Check sheet for the modelled part. Datum: model origin and axes. Units: mm. A direction names the side the tool comes from. Give positions to 0.01 mm unless a question says otherwise; leave off trailing zeros. Write each loop counter-clockwise with the first axis right and the second up, starting at its lowest first coordinate (ties: lowest second). Pieces come first, ordered by that corner, then holes. Notation, with made-up numbers: M -31,71.5 L -14,71.5 A17 ccw -14,78.5 Z; hole C 29.5,30.5 d6. An arc over 180 degrees is marked long. Use CSV: the item, a comma, the result in double quotes. Start each with the question number.
1. Scan lines: line 1 (Y direction, x = 6, z = 48); line 2 (X direction, y = 0, z = 40.5). Record each from-to range of solid material in increasing order.
2. Depth check by flat-ended pin: P1, Ø6, axis at x = -1, z = 45, coming from the -Y side; P2, Ø12, axis at y = 1, z = 43, coming from the +X side; P3, Ø2.5, axis at x = -1, z = 30.5, coming from the -Y side; P4, Ø0.5, axis at x = -4, z = 28.5, coming from the -Y side. Enter the tip coordinate at first touch or a pass-through.
3. Cross-section at A-A, the plane x = -6.5. Enter the section's corners in (y, z).
4. Mould release check, pull along Y, two halves, no side actions. Record for faces 5 (the face through (7, 10, 30)), 6 (the face through (9.15, 8, 30)), 7 (the face through (0, -3, 50)): +Y half, -Y half, draft (parallel to the pull), parting line (faces both ways), or undercut.
5. Access from +Z, -Z, +X, -X, +Y, -Y to the whole of each face (thin tool, end or side, straight path). Record for faces 1 (the face through (-3.967, -9.051, 29.72)), 2 (the face through (-9.051, -3.967, 29.72)), 3 (the face through (4.67, 3.82, 29.72)), 4 (the face through (-10, 7, 30)).
6. Cross-section at D-D, the plane z = 14. State how many separate pieces and enclosed holes the cut face has, and give its area (3 significant figures).
7. Cross-section at B-B, the plane y = 0. Enter the section's corners in (x, z).
Autodesk Inventor part; units mm, degrees
ref_plane "Начальная плоскость" through (0, 0, 10) normal (0, 0, 1) x (1, 0, 0)
ref_plane "Конечная плоскость" through (0, 0, 50) normal (0, 0, 1) x (1, 0, 0)
ref_plane "РабПлоскость4" through (-8.5, 255, 50) normal (0, 0, 1) x (1, 0, 0)
ref_plane "Начальная плоскость" through (0, 0, 10) normal (0, 0, 1) x (1, 0, 0)
ref_plane "Конечная плоскость" through (0, 0, 50) normal (0, 0, 1) x (1, 0, 0)
sketch "Эскиз" plane through (0, 0, 0) normal (0, 0, 1) x (1, 0, 0)
  line L0 (-14.4349, 0) -> (14.4349, 0)
  line L1 (0, -14) -> (0, 14)
  line L2 (0, 0) -> (7.5, 7.5) construction
  circle A0 centre (7.5, 7.5) radius 1.65 construction
  line L3 (5.85, 9.15) -> (9.15, 9.15)
  line L4 (9.15, 9.15) -> (9.15, 5.85)
  line L5 (9.15, 5.85) -> (5.85, 5.85)
  line L6 (5.85, 5.85) -> (5.85, 9.15)
  line L7 (3.235, 8.1636) -> (4.72, 9.9636)
  line L8 (4.7971, 10) -> (8.5, 10)
  line L9 (3.3121, 8) -> (4.95, 8)
  line L10 (4.95, 8) -> (4.95, 5.7985)
  line L11 (4.95, 5.7985) -> (2.6515, 3.5)
  line L12 (0, 3.5) -> (2.6515, 3.5)
  circle A1 centre (0, 0) radius 2.5
  line L13 (8.1636, 3.235) -> (9.9636, 4.72)
  line L14 (10, 4.7971) -> (10, 8.5)
  line L15 (8, 3.3121) -> (8, 4.95)
  line L16 (8, 4.95) -> (5.7985, 4.95)
  line L17 (5.7985, 4.95) -> (3.5, 2.6515)
  line L18 (3.5, 0) -> (3.5, 2.6515)
  arc A2 (10, 8.5) -> (8.5, 10) centre (8.5, 8.5) ccw
  line L19 (0, 0) -> (-7.5, 7.5) construction
  circle A3 centre (-7.5, 7.5) radius 1.65 construction
  line L20 (-5.85, 9.15) -> (-9.15, 9.15)
  line L21 (-9.15, 9.15) -> (-9.15, 5.85)
  line L22 (-9.15, 5.85) -> (-5.85, 5.85)
  line L23 (-5.85, 5.85) -> (-5.85, 9.15)
  line L24 (-3.235, 8.1636) -> (-4.72, 9.9636)
  line L25 (-4.7971, 10) -> (-8.5, 10)
  line L26 (-3.3121, 8) -> (-4.95, 8)
  line L27 (-4.95, 8) -> (-4.95, 5.7985)
  line L28 (-4.95, 5.7985) -> (-2.6515, 3.5)
  line L29 (0, 3.5) -> (-2.6515, 3.5)
  line L30 (-3.5, 0) -> (-3.5, 2.6515)
  line L31 (-5.7985, 4.95) -> (-3.5, 2.6515)
  line L32 (-8, 4.95) -> (-5.7985, 4.95)
  line L33 (-8, 3.3121) -> (-8, 4.95)
  line L34 (-8.1636, 3.235) -> (-9.9636, 4.72)
  line L35 (-10, 4.7971) -> (-10, 8.5)
  arc A4 (-8.5, 10) -> (-10, 8.5) centre (-8.5, 8.5) ccw
  line L36 (0, 14) -> (0, -14)
  line L37 (0, 0) -> (7.5, -7.5) construction
  circle A5 centre (7.5, -7.5) radius 1.65 construction
  line L38 (5.85, -9.15) -> (9.15, -9.15)
  line L39 (9.15, -9.15) -> (9.15, -5.85)
  line L40 (9.15, -5.85) -> (5.85, -5.85)
  line L41 (5.85, -5.85) -> (5.85, -9.15)
  line L42 (3.235, -8.1636) -> (4.72, -9.9636)
  line L43 (4.7971, -10) -> (8.5, -10)
  line L44 (3.3121, -8) -> (4.95, -8)
  line L45 (4.95, -8) -> (4.95, -5.7985)
  line L46 (4.95, -5.7985) -> (2.6515, -3.5)
  line L47 (0, -3.5) -> (2.6515, -3.5)
  line L48 (3.5, 0) -> (3.5, -2.6515)
  line L49 (5.7985, -4.95) -> (3.5, -2.6515)
  line L50 (8, -4.95) -> (5.7985, -4.95)
  line L51 (8, -3.3121) -> (8, -4.95)
  line L52 (8.1636, -3.235) -> (9.9636, -4.72)
  line L53 (10, -4.7971) -> (10, -8.5)
  arc A6 (8.5, -10) -> (10, -8.5) centre (8.5, -8.5) ccw
  line L54 (0, 0) -> (-7.5, -7.5) construction
  line L55 (-4.95, -8) -> (-4.95, -5.7985)
  line L56 (-3.3121, -8) -> (-4.95, -8)
  line L57 (-5.7985, -4.95) -> (-3.5, -2.6515)
  line L58 (-4.95, -5.7985) -> (-2.6515, -3.5)
  line L59 (-3.5, 0) -> (-3.5, -2.6515)
  line L60 (0, -3.5) -> (-2.6515, -3.5)
  circle A7 centre (-7.5, -7.5) radius 1.65 construction
  line L61 (-5.85, -5.85) -> (-5.85, -9.15)
  line L62 (-5.85, -9.15) -> (-9.15, -9.15)
  line L63 (-9.15, -9.15) -> (-9.15, -5.85)
  line L64 (-9.15, -5.85) -> (-5.85, -5.85)
  line L65 (-3.235, -8.1636) -> (-4.72, -9.9636)
  line L66 (-8, -4.95) -> (-5.7985, -4.95)
  line L67 (-8, -3.3121) -> (-8, -4.95)
  line L68 (-8.1636, -3.235) -> (-9.9636, -4.72)
  line L69 (-4.7971, -10) -> (-8.5, -10)
  line L70 (-10, -4.7971) -> (-10, -8.5)
  arc A8 (-10, -8.5) -> (-8.5, -10) centre (-8.5, -8.5) ccw
  arc A9 (3.235, 8.1636) -> (3.3121, 8) centre (3.3121, 8.1) ccw
  arc A10 (4.7971, 10) -> (4.72, 9.9636) centre (4.7971, 9.9) ccw
  arc A11 (8, 3.3121) -> (8.1636, 3.235) centre (8.1, 3.3121) ccw
  arc A12 (9.9636, 4.72) -> (10, 4.7971) centre (9.9, 4.7971) ccw
  arc A13 (-3.3121, 8) -> (-3.235, 8.1636) centre (-3.3121, 8.1) ccw
  arc A14 (-4.72, 9.9636) -> (-4.7971, 10) centre (-4.7971, 9.9) ccw
  arc A15 (-8.1636, 3.235) -> (-8, 3.3121) centre (-8.1, 3.3121) ccw
  arc A16 (-10, 4.7971) -> (-9.9636, 4.72) centre (-9.9, 4.7971) ccw
  arc A17 (-8, -3.3121) -> (-8.1636, -3.235) centre (-8.1, -3.3121) ccw
  arc A18 (-9.9636, -4.72) -> (-10, -4.7971) centre (-9.9, -4.7971) ccw
  arc A19 (-3.235, -8.1636) -> (-3.3121, -8) centre (-3.3121, -8.1) ccw
  arc A20 (-4.7971, -10) -> (-4.72, -9.9636) centre (-4.7971, -9.9) ccw
  arc A21 (4.72, -9.9636) -> (4.7971, -10) centre (4.7971, -9.9) ccw
  arc A22 (3.3121, -8) -> (3.235, -8.1636) centre (3.3121, -8.1) ccw
  arc A23 (8.1636, -3.235) -> (8, -3.3121) centre (8.1, -3.3121) ccw
  arc A24 (10, -4.7971) -> (9.9636, -4.72) centre (9.9, -4.7971) ccw
  point P0 (3.1, 8)
  point P1 (4.75, 10)
  point P2 (7.5, 9.15)
  point P3 (8, 3.1)
  point P4 (10, 4.75)
  point P5 (7.5, 5.85)
  point P6 (9.15, 7.5)
  point P7 (-3.1, 8)
  point P8 (-4.75, 10)
  point P9 (-7.5, 9.15)
  point P10 (-8, 3.1)
  point P11 (-10, 4.75)
  point P12 (-7.5, 5.85)
  point P13 (-9.15, 7.5)
  point P14 (3.1, -8)
  point P15 (4.75, -10)
  point P16 (7.5, -9.15)
  point P17 (8, -3.1)
  point P18 (10, -4.75)
  point P19 (7.5, -5.85)
  point P20 (9.15, -7.5)
  point P21 (-3.1, -8)
  point P22 (-7.5, -5.85)
  point P23 (-7.5, -9.15)
  point P24 (-9.15, -7.5)
  point P25 (-4.75, -10)
  point P26 (-8, -3.1)
  point P27 (-10, -4.75)
  dimension "d0" = 45
  dimension "d1" = 3.3
  dimension "d2" = 1.5
  dimension "d3" = 1.2
  dimension "d4" = 5
  dimension "d5" = 6.5
  dimension "d6" = 15
  dimension "d7" = 20
  dimension "d8" = 9.9
  dimension "d9" = 9.5
  dimension "d10" = 6.2
  dimension "d11" = 2
  dimension "d18" = 0.1
  dimension "d19" = 0.1
extrude "Тело" add sketch "Эскиз" along normal up to surface (40 mm away) from surface at 10 contours A1 L1 L12 L11 L10 L9 A9 L7 A10 L8 A2 L14 A12 L13 A11 L15 L16 L17 L18 L0 | L0 L48 L49 L50 L51 A23 L52 A24 L53 A6 L43 A21 L42 A22 L44 L45 L46 L47 L1 A1 | A1 L0 L30 L31 L32 L33 A15 L34 A16 L35 A4 L25 A14 L24 A13 L26 L27 L28 L29 L1 | L1 L60 L58 L55 L56 A19 L65 A20 L69 A8 L70 A18 L68 A17 L67 L66 L57 L59 L0 A1
sketch "Эскиз2" plane through (0, 0, 0) normal (0, 0, 1) x (1, 0, 0)
  line L0 (0, 0) -> (10, 0)
ref_plane "РабПлоскость3" through (0, 0, 0) normal (0, -1, 0) x (1, 0, 0)
sketch "Эскиз3" plane through (0, 0, 0) normal (0, -1, 0) x (1, 0, 0)
  line L0 (-2, 10) -> (12, 10)
  line L1 (-2, 50) -> (12, 50)
  dimension "d25" = 40
ref_plane "РабПлоскость4" through (-8.5, 255, 50) normal (0, 0, 1) x (1, 0, 0)
split "Разделение1" plane through (-8.5, 255, 50) removes the side toward (0, 0, 1)
ref_plane "РабПлоскость5" through (4.7971, -255, 10) normal (0, 0, -1) x (-1, 0, 0)
split "Разделение2" plane through (4.7971, -255, 10) removes the side toward (0, 0, -1)
properties part number "короткая палка"
Worked answers:
1,line 1,"y = -10 to -9.15, -5.85 to -4.95, 4.95 to 5.85, 9.15 to 10"
1,line 2,"x = -3.5 to -2.5, 2.5 to 3.5"
2,P1,"stops at y = -9.09"
2,P2,"stops at x = 10"
2,P3,"stops at y = -3.5"
2,P4,"stops at y = -9.39"
3,outline,"M -10,10 L -9.15,10 L -9.15,50 L -10,50 Z; M -5.85,10 L -4.95,10 L -4.95,50 L -5.85,50 Z; M 4.95,10 L 5.85,10 L 5.85,50 L 4.95,50 Z; M 9.15,10 L 10,10 L 10,50 L 9.15,50 Z"
4,face 5,"+Y half"
4,face 6,"undercut"
4,face 7,"draft"
5,face 1,"+Z, -Z, -Y"
5,face 2,"+Z, -Z, -X"
5,face 3,"+Z, -Z"
5,face 4,"+Z, -Z, -X, +Y, -Y"
6,separate pieces,"1"
6,enclosed holes,"5"
6,area,"115 mm^2"
7,outline,"M -3.5,10 L -2.5,10 L -2.5,50 L -3.5,50 Z; M 2.5,10 L 3.5,10 L 3.5,50 L 2.5,50 Z"
